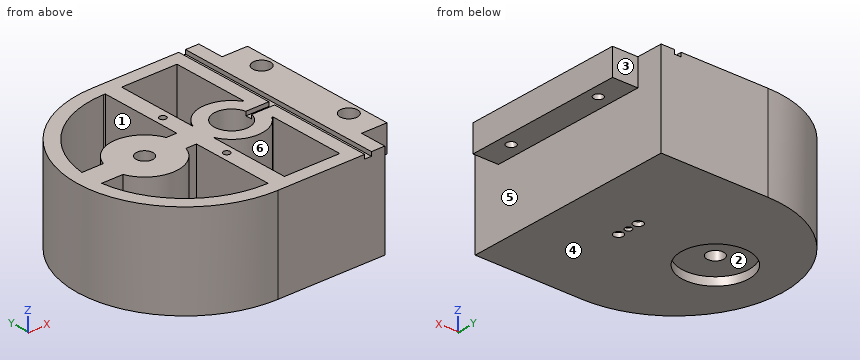
Autodesk Inventor part; units mm, degrees
ref_plane "YZ Plane" through (0, 0, 0) normal (1, 0, 0) x (0, 1, 0)
ref_plane "XZ Plane" through (0, 0, 0) normal (0, 1, 0) x (-1, 0, 0)
ref_plane "XY Plane" through (0, 0, 0) normal (0, 0, 1) x (1, 0, 0)
sketch "Sketch1" plane through (0, 0, 0) normal (0, 0, 1) x (1, 0, 0)
  line L0 (0, 0) -> (160, 0)
  line L1 (160, 0) -> (160, 160)
  line L2 (160, 160) -> (0, 160)
  line L3 (0, 160) -> (0, 0)
  circle A0 centre (50, 80) radius 6.25
  point P0 (160, 80)
  dimension "d0" = 160
  dimension "d1" = 160
  dimension "d2" = 12.5
  dimension "d7" = 50
extrude "Extrusion1" add sketch "Sketch1" along normal blind 70
sketch "Sketch2" plane through (0, 0, 70) normal (0, 0, 1) x (1, 0, 0)
  circle A0 centre (115, 80) radius 2.5
  line L0 (160, 0) -> (160, 160)
  circle A1 centre (50, 80) radius 6.25
  line L1 (0, 0) -> (160, 0)
  line L2 (160, 0) -> (160, 160)
  line L3 (160, 160) -> (0, 160)
  line L4 (0, 160) -> (0, 0)
  point P0 (160, 80)
  dimension "d8" = 5
  dimension "d9" = 65
extrude "Extrusion2" cut sketch "Sketch2" against normal through all contours A0
sketch "Sketch5" plane through (0, 0, 70) normal (0, 0, 1) x (1, 0, 0)
  circle A0 centre (50, 80) radius 6.25
  line L0 (0, 0) -> (160, 0)
  line L1 (160, 0) -> (160, 160)
  line L2 (160, 160) -> (0, 160)
  line L3 (0, 160) -> (0, 0)
  circle A1 centre (80, 80) radius 80 construction
  line L4 (0, 0) -> (160, 0)
  arc A2 (80, 160) -> (80, 0) centre (80, 80) ccw
  line L5 (160, 160) -> (0, 160)
  line L6 (80, 160) -> (0, 160)
  line L7 (0, 160) -> (0, 0)
  line L8 (80, 0) -> (0, 0)
  point P0 (0, 80)
extrude "Extrusion5" cut sketch "Sketch5" against normal through all contours L3 A2 L0 | L3 L2 A2
sketch "Sketch21" plane through (0, 0, 70) normal (0, 0, 1) x (1, 0, 0)
  circle A0 centre (115, 80) radius 2.5
  circle A1 centre (115, 80) radius 13
  point P0 (0, 0)
  dimension "d100" = 26
extrude "Extrusion21" cut sketch "Sketch21" against normal blind 65
sketch "Sketch22" plane through (115, 80, 5) normal (0, 0, 1) x (1, 0, 0)
  circle A0 centre (0, 8.5) radius 2
  circle A1 centre (0, -8.5) radius 2
  circle A2 centre (0, 0) radius 2.5 construction
  line L0 (0, 8.5) -> (0, -8.5) construction
  point P0 (-115, -80)
  dimension "d103" = 4
  dimension "d104" = 4
  dimension "d105" = 17
extrude "Extrusion22" cut sketch "Sketch22" against normal through all
sketch "Sketch23" plane through (0, 0, 0) normal (0, 0, -1) x (-1, 0, 0)
  circle A0 centre (-115, 88.5) radius 2
  circle A1 centre (-115, 71.5) radius 2
  circle A2 centre (-115, 88.5) radius 3.5
  circle A3 centre (-115, 71.5) radius 3.5
  point P0 (0, 0)
  dimension "d108" = 7
  dimension "d109" = 7
extrude "Extrusion23" cut sketch "Sketch23" against normal blind 3 contours A0 | A1 | A2 | A3
sketch "Sketch24" plane through (115, 80, 5) normal (0, 0, 1) x (1, 0, 0)
  circle A0 centre (0, 0) radius 2.5
  circle A1 centre (0, 0) radius 4
  point P0 (-115, -80)
  dimension "d112" = 8
extrude "Extrusion24" cut sketch "Sketch24" against normal blind 3
sketch "Sketch25" plane through (0, 0, 70) normal (0, 0, 1) x (1, 0, 0)
  line L0 (115, 77.5) -> (150, 77.5)
  line L1 (150, 77.5) -> (150, 82.5)
  line L2 (150, 82.5) -> (115, 82.5)
  line L3 (115, 82.5) -> (115, 77.5)
  line L4 (160, 0) -> (160, 160)
  line L5 (80, 0) -> (160, 0)
  line L6 (160, 160) -> (80, 160)
  line L7 (150, 0) -> (145, 0)
  line L8 (145, 0) -> (145, 160)
  line L9 (145, 160) -> (150, 160)
  line L10 (150, 160) -> (150, 0)
  point P0 (0, 0)
  point P1 (115, 88.5)
  point P2 (150, 80)
  point P3 (160, 80)
  dimension "d115" = 10
  dimension "d116" = 5
  dimension "d119" = 5
extrude "Extrusion25" cut sketch "Sketch25" against normal blind 3 contours L3 L2 L8 L0 | L8 L2 L1 L0 | L0 L10 L5 L8 | L8 L6 L10 L2
sketch "Sketch26" plane through (0, 0, 70) normal (0, 0, 1) x (1, 0, 0)
  line L0 (160, 0) -> (160, 160)
  line L1 (160, 20) -> (179, 20)
  line L2 (179, 20) -> (179, 140)
  line L3 (179, 140) -> (160, 140)
  line L4 (160, 140) -> (160, 20)
  line L5 (80, 0) -> (145, 0)
  line L6 (145, 160) -> (80, 160)
  circle A0 centre (170, 42.5) radius 3.5
  line L7 (170, 117.5) -> (170, 42.5) construction
  circle A1 centre (170, 117.5) radius 3.5
  point P0 (0, 0)
  point P1 (179, 80)
  point P2 (170, 80)
  dimension "d120" = 19
  dimension "d121" = 20
  dimension "d122" = 20
  dimension "d123" = 7
  dimension "d124" = 10
  dimension "d142" = 75
  dimension "d143" = 7
extrude "Extrusion26" add sketch "Sketch26" against normal blind 20
sketch "Sketch27" plane through (0, 0, 70) normal (0, 0, 1) x (1, 0, 0)
  line L0 (179, 52.5) -> (87.5, 52.5) construction
  line L1 (87.5, 52.5) -> (87.5, 107.5) construction
  line L2 (87.5, 107.5) -> (179, 107.5) construction
  line L3 (179, 107.5) -> (179, 52.5) construction
  line L4 (179, 20) -> (179, 140) construction
  circle A0 centre (87.5, 52.5) radius 2.5
  circle A1 centre (87.5, 107.5) radius 2.5
  point P0 (0, 0)
  point P1 (179, 80)
  dimension "d127" = 91.5
  dimension "d128" = 55
  dimension "d129" = 5
  dimension "d130" = 5
extrude "Extrusion27" cut sketch "Sketch27" against normal blind 25
sketch "Sketch28" plane through (0, 0, 0) normal (0, 0, -1) x (-1, 0, 0)
  circle A0 centre (-50, 80) radius 25
  circle A1 centre (-50, 80) radius 6.25
  point P0 (0, 0)
  dimension "d133" = 50
extrude "Extrusion28" cut sketch "Sketch28" against normal blind 6 contours A0 | A1
sketch "Sketch29" plane through (0, 0, 70) normal (0, 0, 1) x (1, 0, 0)
  circle A0 centre (170, 42.5) radius 3.5
  circle A1 centre (170, 42.5) radius 6.5
  circle A2 centre (170, 117.5) radius 3.5
  circle A3 centre (170, 117.5) radius 6.5
  point P0 (0, 0)
  dimension "d136" = 13
  dimension "d144" = 13
extrude "Extrusion29" cut sketch "Sketch29" against normal blind 15 contours A0 | A1 | A3
sketch "Sketch30" plane through (0, 0, 70) normal (0, 0, 1) x (1, 0, 0)
  circle A0 centre (87.5, 52.5) radius 2.5
  circle A1 centre (87.5, 107.5) radius 2.5
  line L0 (145, 82.5) -> (145, 160)
  line L1 (145, 160) -> (80, 160)
  arc A2 (80, 160) -> (80, 0) centre (80, 80) ccw
  line L2 (80, 0) -> (145, 0)
  line L3 (145, 0) -> (145, 77.5)
  line L4 (145, 77.5) -> (127.7574, 77.5)
  arc A3 (127.7574, 82.5) -> (127.7574, 77.5) centre (115, 80) ccw
  line L5 (127.7574, 82.5) -> (145, 82.5)
  circle A4 centre (50, 80) radius 6.25 construction
  circle A5 centre (50, 80) radius 25 construction
  circle A6 centre (115, 88.5) radius 3.5
  circle A7 centre (115, 71.5) radius 3.5
  arc A8 (80, 160) -> (80, 0) centre (80, 80) ccw
  line L6 (160, 160) -> (80, 160)
  line L7 (160, 0) -> (160, 160)
  line L8 (80, 0) -> (160, 0)
  circle A9 centre (115, 80) radius 2.5
  arc A10 (80, 150) -> (80, 10) centre (80, 80) ccw construction
  line L9 (80, 150) -> (135, 150) construction
  line L10 (135, 150) -> (135, 92.5)
  line L11 (135, 92.5) -> (134.3067, 92.5)
  arc A11 (134.3067, 92.5) -> (134.3067, 67.5) centre (115, 80) ccw construction
  line L12 (134.3067, 67.5) -> (135, 67.5)
  line L13 (135, 67.5) -> (135, 10)
  line L14 (135, 10) -> (80, 10) construction
  line L15 (93.6283, 71.5) -> (10.518, 71.5) construction
  line L16 (93.6283, 88.5) -> (10.518, 88.5) construction
  arc A12 (80, 150) -> (10.518, 88.5) centre (80, 80) ccw
  arc A13 (10.518, 71.5) -> (80, 10) centre (80, 80) ccw
  arc A14 (134.3067, 92.5) -> (93.6283, 88.5) centre (115, 80) ccw
  arc A15 (93.6283, 71.5) -> (134.3067, 67.5) centre (115, 80) ccw
  line L17 (81.3717, 150) -> (81.3717, 10) construction
  line L18 (93.6283, 88.5) -> (93.6283, 150)
  line L19 (93.6283, 71.5) -> (93.6283, 10)
  line L20 (87.5, 52.5) -> (87.5, 107.5) construction
  line L21 (80, 150) -> (81.3717, 150)
  line L22 (80, 10) -> (81.3717, 10)
  line L23 (93.6283, 10) -> (135, 10)
  line L24 (93.6283, 150) -> (135, 150)
  line L25 (81.3717, 150) -> (81.3717, 88.5)
  line L26 (81.3717, 71.5) -> (81.3717, 10)
  line L27 (10.518, 71.5) -> (81.3717, 71.5) construction
  line L28 (10.518, 88.5) -> (81.3717, 88.5) construction
  line L29 (10.518, 88.5) -> (26.4894, 88.5)
  circle A16 centre (50, 80) radius 25 construction
  line L30 (10.518, 71.5) -> (26.4894, 71.5)
  line L31 (81.3717, 71.5) -> (73.5106, 71.5)
  line L32 (81.3717, 88.5) -> (73.5106, 88.5)
  arc A17 (73.5106, 88.5) -> (26.4894, 88.5) centre (50, 80) ccw
  arc A18 (26.4894, 71.5) -> (73.5106, 71.5) centre (50, 80) ccw
  point P0 (0, 0)
  dimension "d139" = 10
extrude "Extrusion30" cut sketch "Sketch30" against normal blind 60 contours L10 L11 A14 L18 L24 | L12 L13 L23 L19 A15 | L21 L25 L32 A17 L29 A12 | L30 A18 L31 L26 L22 A13
properties part number "AA005b" material "ABS Plastic"
CAD build for the part. Positions are in the model's coordinates, mm. Face numbers are marked on the shaded views. A direction names the side the tool comes from. Coordinates: 2 decimals unless noted, no trailing zeros. Order: outer loops, then holes, each group sorted by start corner. A loop starts at its lowest first (then second) coordinate and runs counter-clockwise, first axis right, second up. Notation, with made-up numbers: M 1.5,17 L 17.5,17 A14 cw 17.5,39 Z; hole C 38.25,-18.75 d8. An arc over 180 degrees is marked long. Answer as CSV lines item,"result".
1) 3-axis set-ups, long thin cutter, end or side, ignore diameter. For the marked faces 1, 2 and 3: which of +Z, -Z, +X, -X, +Y, -Y reach the whole face in a straight line?
Verdict:
face 1,"+Z"
face 2,"-Z"
face 3,"+Z, -Z, +X, +Y"
2) Cut at D-D (y = 52.5). List the corners of the cut face in (x, z), then the cut area to 3 significant figures.
Verdict:
outline,"M 4.88,0 L 160,0 L 160,50 L 179,50 L 179,70 L 150,70 L 150,67 L 145,67 L 145,70 L 135,70 L 135,10 L 93.63,10 L 93.63,70 L 90,70 L 90,45 L 85,45 L 85,70 L 81.37,70 L 81.37,10 L 15.63,10 L 15.63,70 L 4.88,70 Z"
area,"4,670 mm2"
3) Flat gauge pins, fed straight in: P1, Ø20.5, axis at x = 118, y = 26.5, coming from the +Z side; P2, Ø20, axis at x = 50, y = 80, coming from the -Z side; P3, Ø11.5, axis at x = 170, y = 42.5, coming from the -Z side. Where does each tip first touch, or does it go through?
Verdict:
P1,"z = 10"
P2,"z = 6"
P3,"z = 50"
4) Mould opens along X. For the marked faces 4, 5 and 6 say: released by +X, released by -X, zero draft, split by the parting line, or undercut.
Verdict:
face 4,"zero draft"
face 5,"released by +X"
face 6,"undercut"
5) Cut at A-A (y = 80). List the corners of the cut face in (x, z).
Verdict:
outline,"M 0,0 L 25,0 L 25,6 L 43.75,6 L 43.75,70 L 0,70 Z; M 56.25,6 L 75,6 L 75,0 L 112.5,0 L 112.5,2 L 111,2 L 111,5 L 102,5 L 102,70 L 56.25,70 Z; M 117.5,0 L 160,0 L 160,50 L 179,50 L 179,70 L 150,70 L 150,67 L 128,67 L 128,5 L 119,5 L 119,2 L 117.5,2 Z"
6) Cut at B-B (z = 26). List the corners of the cut face in (x, y).
Verdict:
outline,"M 80,0 L 160,0 L 160,160 L 80,160 A80 ccw Z; hole M 10.52,71.5 A70 ccw 80,10 L 81.37,10 L 81.37,71.5 L 73.51,71.5 A25 cw 26.49,71.5 Z; hole M 10.52,88.5 L 26.49,88.5 A25 cw 73.51,88.5 L 81.37,88.5 L 81.37,150 L 80,150 A70 ccw Z; hole C 50,80 d12.5; hole M 93.63,10 L 135,10 L 135,67.5 L 134.31,67.5 A23 cw 93.63,71.5 Z; hole M 93.63,88.5 A23 cw 134.31,92.5 L 135,92.5 L 135,150 L 93.63,150 Z; hole C 115,80 d26"
7) Cut at C-C (x = 65.5). List the corners of the cut face in (y, z) (3 decimals), then the cut area to 3 significant figures.
Verdict:
outline,"M 1.325,0 L 60.385,0 L 60.385,6 L 99.615,6 L 99.615,0 L 158.675,0 L 158.675,70 L 148.482,70 L 148.482,10 L 99.615,10 L 99.615,70 L 60.385,70 L 60.385,10 L 11.518,10 L 11.518,70 L 1.325,70 Z"
area,"4,920 mm2"
8) Drill centre lines: L1, parallel to Y at x = 115, z = 3.75; L2, parallel to Y at x = 170, z = 60.5; L3, parallel to Y at x = 87, z = 51. Where is each one in solid material? Low to high. Write a range as from..to.
Verdict:
L1,"0..69.5, 73.5..76, 84..86.5, 90.5..160"
L2,"20..36, 49..111, 124..140"
L3,"0..50.05, 54.95..105.05, 109.95..160"
